Could you check a few things on this model? Use its own coordinates, in mm. Give positions to 0.01 mm unless a question says otherwise; leave off trailing zeros. Order: outer loops, then holes, each group sorted by start corner. A loop starts at its lowest first (then second) coordinate and runs counter-clockwise, first axis right, second up.
(1) Imagine slicing it at D-D, the plane z = -16.7. Write out the boundary of the cut face in (x, y), then the cut area to 3 significant figures.
(2) Imagine slicing it at C-C, the plane y = 0.45. State how many separate pieces and enclosed holes the cut face has, then the cut area to 3 significant figures.
(3) Imagine slicing it at A-A, the plane z = 0. Write out the boundary of the cut face in (x, y), then the cut area to 3 significant figures.
(4) If I drill on probe 1 along X at (y, z) = (1.55, 0); probe 2 along Z at (x, y) = (-28, 1.65); probe 3 along X at (y, z) = (2.1, -27.5), over which ranges is the centre line in solid material (lowest first)?
(5) Will these pins go through, and if not, where does the flat tip stop? pin 1 (1.5 mm diameter, centred on x = -26.5, y = 1.5, fed in from +Z); pin 2 (1.5 mm diameter, centred on x = -25, y = 2, fed in from +Z); pin 3 (19.5 mm diameter, centred on x = 0, z = -26.84, fed in from -Y); pin 4 (1.5 mm diameter, centred on y = 0.5, z = -16, fed in from -X).
(6) Imagine slicing it at B-B, the plane x = 0. Write out the boundary of the cut face in (y, z), then the cut area to 3 significant figures.
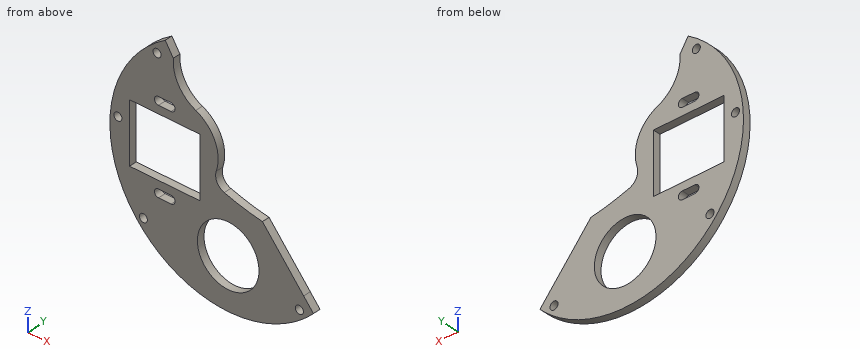
from build123d import *

# Parameters (mm, degrees)
SKETCH1_R           = 12.247413434
SKETCH1_R_2         = 1.6
BOSS_EXTRUDE1_DEPTH = 3


with BuildPart() as part:
    # Sketch1 → Boss-Extrude1 (new body)
    # profile 1 of 4: a face of its own
    with BuildSketch(Plane(origin=(0, 0, 0), x_dir=(1, 0, 0), z_dir=(0, 1, 0))):
        with BuildLine():
            ThreePointArc((-1.570198622, 4.747049219), (5.939862085, 6.896641641), (13.599748073, 8.42892949))
            Line((13.599748073, 8.42892949), (29.987808283, 27.959459121))
            Line((29.987808283, 27.959459121), (33.869799276, 32.585835834))
            ThreePointArc((33.869799276, 32.585835834), (30.211017655, 36.004088827), (26.209354845, 39.013711931))
            Line((26.209354845, 39.013711931), (22.327363852, 34.387335218))
            ThreePointArc((22.327363852, 34.387335218), (-14.018145326, 38.529100711), (-39.204591568, 12))
            Line((-39.204591568, 12), (-11.204591568, 12))
            Line((-11.204591568, 12), (-11.204591568, -12))
            Line((-11.204591568, -12), (-39.204591568, -12))
            ThreePointArc((-39.204591568, -12), (-32.558798287, -24.918359779), (-21.825227783, -34.708204106))
            ThreePointArc((-21.825227783, -34.708204106), (-19.713839088, -25.875293038), (-12.892481496, -19.879681247))
            ThreePointArc((-12.892481496, -19.879681247), (-5.276324008, -12.302707641), (-4.746257371, -1.572590527))
            ThreePointArc((-4.746257371, -1.572590527), (-4.467534634, 2.245247045), (-1.570198622, 4.747049219))
        make_face()
        with BuildLine():
            Line((-22.704591568, -18.3), (-27.704591568, -18.3))
            ThreePointArc((-27.704591568, -18.3), (-29.304591568, -16.7), (-27.704591568, -15.1))
            Line((-27.704591568, -15.1), (-22.704591568, -15.1))
            ThreePointArc((-22.704591568, -15.1), (-21.104591568, -16.7), (-22.704591568, -18.3))
        make_face(mode=Mode.SUBTRACT)
        with BuildLine():
            ThreePointArc((-27.704591568, 15.1), (-29.304591568, 16.7), (-27.704591568, 18.3))
            Line((-27.704591568, 18.3), (-22.704591568, 18.3))
            ThreePointArc((-22.704591568, 18.3), (-21.104591568, 16.7), (-22.704591568, 15.1))
            Line((-22.704591568, 15.1), (-27.704591568, 15.1))
        make_face(mode=Mode.SUBTRACT)
        with Locations(Location((0, 26.835034763, 0), (0, 0, 270))):
            Circle(SKETCH1_R, mode=Mode.SUBTRACT)
        with Locations(Location((28.282654826, 33.705955497, 0), (0, 0, 270))):
            Circle(SKETCH1_R_2, mode=Mode.SUBTRACT)
    # profile 2 of 4: a face of its own
    with BuildSketch(Plane(origin=(0, 0, 0), x_dir=(1, 0, 0), z_dir=(0, 1, 0))):
        with BuildLine():
            Line((-25.019163556, -39.787453487), (-21.825227783, -34.708204106))
            ThreePointArc((-21.825227783, -34.708204106), (-32.558798287, -24.918359779), (-39.204591568, -12))
            ThreePointArc((-39.204591568, -12), (-41, 0), (-39.204591568, 12))
            ThreePointArc((-39.204591568, 12), (-14.018145326, 38.529100711), (22.327363852, 34.387335218))
            Line((22.327363852, 34.387335218), (26.209354845, 39.013711931))
            ThreePointArc((26.209354845, 39.013711931), (-39.405076534, 25.617180629), (-25.019163556, -39.787453487))
        make_face()
        with Locations(Location((-28.282654826, -33.705955497, 0), (0, 0, 270))):
            Circle(SKETCH1_R_2, mode=Mode.SUBTRACT)
        with Locations(Location((-43.832566716, -3.834852681, 0), (0, 0, 270))):
            Circle(SKETCH1_R_2, mode=Mode.SUBTRACT)
        with Locations(Location((-33.705955497, 28.282654826, 0), (0, 0, 270))):
            Circle(SKETCH1_R_2, mode=Mode.SUBTRACT)
    # profile 3 of 4: a face of its own
    with BuildSketch(Plane(origin=(0, 0, 0), x_dir=(1, 0, 0), z_dir=(0, 1, 0))):
        with BuildLine():
            ThreePointArc((-39.204591568, 12), (-41, 0), (-39.204591568, -12))
            Line((-39.204591568, -12), (-39.204591568, 12))
        make_face()
    # profile 4 of 4: a face of its own
    with BuildSketch(Plane(origin=(0, 0, 0), x_dir=(1, 0, 0), z_dir=(0, 1, 0))):
        with BuildLine():
            ThreePointArc((-1.570198622, 4.747049219), (5.939862085, 6.896641641), (13.599748073, 8.42892949))
            Line((13.599748073, 8.42892949), (29.987808283, 27.959459121))
            Line((29.987808283, 27.959459121), (33.869799276, 32.585835834))
            ThreePointArc((33.869799276, 32.585835834), (30.211017655, 36.004088827), (26.209354845, 39.013711931))
            Line((26.209354845, 39.013711931), (22.327363852, 34.387335218))
            ThreePointArc((22.327363852, 34.387335218), (-14.018145326, 38.529100711), (-39.204591568, 12))
            Line((-39.204591568, 12), (-11.204591568, 12))
            Line((-11.204591568, 12), (-11.204591568, -12))
            Line((-11.204591568, -12), (-39.204591568, -12))
            ThreePointArc((-39.204591568, -12), (-32.558798287, -24.918359779), (-21.825227783, -34.708204106))
            ThreePointArc((-21.825227783, -34.708204106), (-19.713839088, -25.875293038), (-12.892481496, -19.879681247))
            ThreePointArc((-12.892481496, -19.879681247), (-5.276324008, -12.302707641), (-4.746257371, -1.572590527))
            ThreePointArc((-4.746257371, -1.572590527), (-4.467534634, 2.245247045), (-1.570198622, 4.747049219))
        make_face()
        with BuildLine():
            Line((-22.704591568, -18.3), (-27.704591568, -18.3))
            ThreePointArc((-27.704591568, -18.3), (-29.304591568, -16.7), (-27.704591568, -15.1))
            Line((-27.704591568, -15.1), (-22.704591568, -15.1))
            ThreePointArc((-22.704591568, -15.1), (-21.104591568, -16.7), (-22.704591568, -18.3))
        make_face(mode=Mode.SUBTRACT)
        with BuildLine():
            ThreePointArc((-27.704591568, 15.1), (-29.304591568, 16.7), (-27.704591568, 18.3))
            Line((-27.704591568, 18.3), (-22.704591568, 18.3))
            ThreePointArc((-22.704591568, 18.3), (-21.104591568, 16.7), (-22.704591568, 15.1))
            Line((-22.704591568, 15.1), (-27.704591568, 15.1))
        make_face(mode=Mode.SUBTRACT)
        with Locations(Location((0, 26.835034763, 0), (0, 0, 270))):
            Circle(SKETCH1_R, mode=Mode.SUBTRACT)
        with Locations(Location((28.282654826, 33.705955497, 0), (0, 0, 270))):
            Circle(SKETCH1_R_2, mode=Mode.SUBTRACT)
    extrude(amount=BOSS_EXTRUDE1_DEPTH)


solid = part.part
Answer block:
1. outline: (-43.93, 0) - (-29.3, 0) - (-29.3, 3) - (-43.93, 3) - close; (-21.1, 0) - (-6.88, 0) - (-6.88, 3) - (-21.1, 3) - close; (6.88, 0) - (20.54, 0) - (20.54, 3) - (6.88, 3) - close
1. area: 128 mm2
2. separate pieces: 1
2. enclosed holes: 8
2. area: 2,510 mm2
3. outline: (-47, 0) - (-39.2, 0) - (-39.2, 3) - (-47, 3) - close; (-11.2, 0) - (-5, 0) - (-5, 3) - (-11.2, 3) - close
3. area: 42.0 mm2
4. probe 1: x = -47 to -39.2, -11.2 to -5
4. probe 2: z = -37.75 to -18.27, -15.13 to -12, 12 to 15.13, 18.27 to 32.13, 35.28 to 37.75
4. probe 3: x = -38.11 to -35.1, -32.31 to -12.23, 12.23 to 29.6
5. pin 1: stops at z = 39.32
5. pin 2: stops at z = 39.79
5. pin 3: passes through
5. pin 4: stops at x = -44.46
6. outline: (0, -47) - (3, -47) - (3, -39.08) - (0, -39.08) - close; (0, -14.59) - (3, -14.59) - (3, -5.25) - (0, -5.25) - close
6. area: 51.8 mm2
